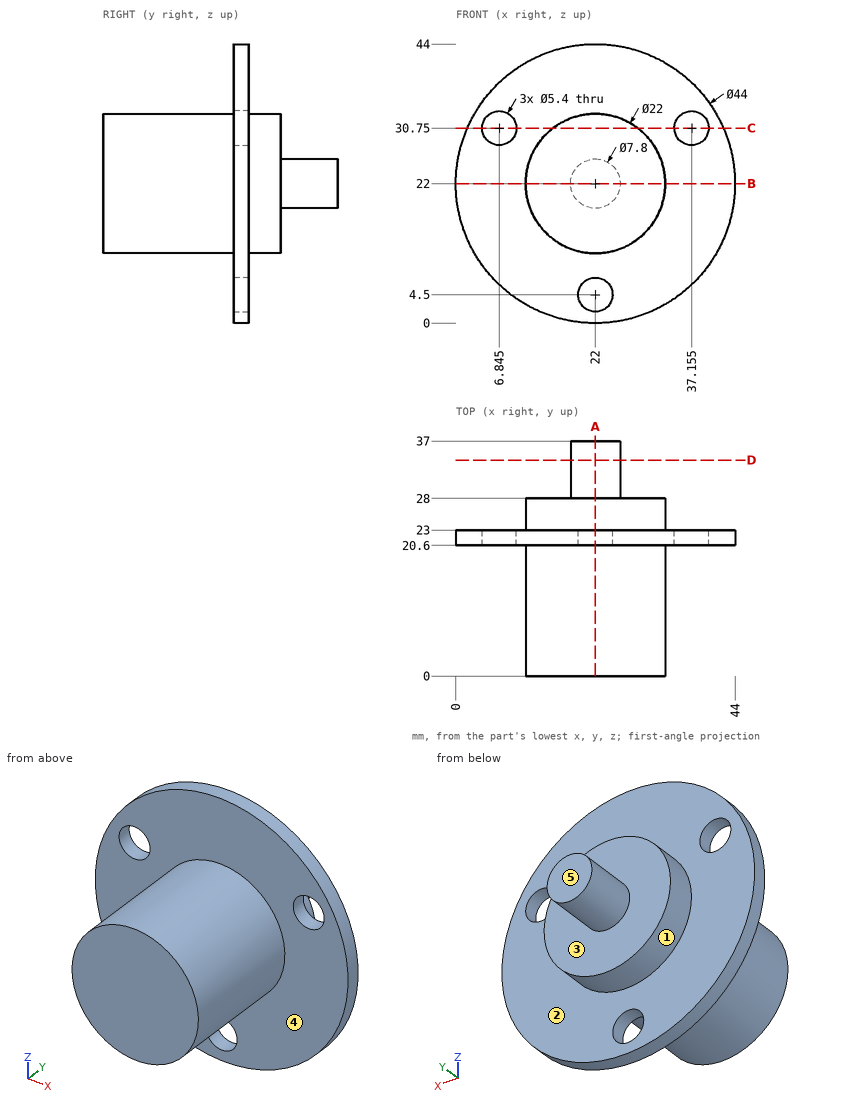
Check sheet for the drawn part. Datum: minimum x, y, z corner. Units: mm. A direction names the side the tool comes from. Round coordinates to 2 decimals unless told otherwise and drop trailing zeros. Loops run counter-clockwise (first coordinate to the right, second up) from the corner with the lowest first, then second, coordinate; pieces in that order, holes last. Notation, with made-up numbers: (89, 31.25) -> (95, 31.25) arc R35 cw to (95, 69.25) -> close; hole circle Ø9 at (28, 48). An arc over 180 degrees is marked (long way). Put each result on its own line as item: value. Start each with the question number.
1. Scan lines: probe 1 along Y at (x, z) = (31, 21); probe 2 along X at (y, z) = (22.4, 30.75) (1 decimal); probe 3 along Y at (x, z) = (27.5, 35.5). Record each from-to range of solid material in increasing order.
2. Section check C-C (z = 30.75). Enter the section's corners in (x, y) (1 decimal), plus the area to 3 significant figures.
3. Gauge pin test, flat ends, axial feed: pin 1 (22 mm diameter, centred on x = 32, z = 15, fed in from +Y); pin 2 (1 mm diameter, centred on x = 34, z = 12, fed in from -Y); pin 3 (1 mm diameter, centred on x = 6.5, z = 7, fed in from +Y); pin 4 (12 mm diameter, centred on x = 32.5, y = 6.5, fed in from -Z). Record the tip position at first contact, or that the pin passes through.
4. Draft check along X on the marked faces 1 and 2. Enter one of: +X half, -X half, draft (parallel to the pull), parting line (faces both ways), or undercut.
5. Section check B-B (z = 22). Enter the section's corners in (x, y).
6. Section check A-A (x = 22). Enter the section's corners in (y, z), plus the area to 3 significant figures.
7. Section check D-D (y = 34). Enter the section's corners in (x, z), plus the area to 3 significant figures.
8. Access from +Z, -Z, +X, -X, +Y, -Y to the whole of each face (thin tool, end or side, straight path). Record for the marked faces 3, 4 and 5.
Findings:
1. probe 1: y = 0 to 28
1. probe 2: x = 1.8 to 4.1, 9.5 to 34.5, 39.9 to 42.2
1. probe 3: y = 20.6 to 23
2. outline: (1.8, 20.6) -> (4.1, 20.6) -> (4.1, 23) -> (1.8, 23) -> close; (9.5, 20.6) -> (15.3, 20.6) -> (15.3, 0) -> (28.7, 0) -> (28.7, 20.6) -> (34.5, 20.6) -> (34.5, 23) -> (28.7, 23) -> (28.7, 28) -> (15.3, 28) -> (15.3, 23) -> (9.5, 23) -> close; (39.9, 20.6) -> (42.2, 20.6) -> (42.2, 23) -> (39.9, 23) -> close
2. area: 412 mm^2
3. pin 1: stops at y = 37
3. pin 2: stops at y = 20.6
3. pin 3: stops at y = 23
3. pin 4: stops at z = 11.96
4. face 1: parting line
4. face 2: draft
5. outline: (0, 20.6) -> (11, 20.6) -> (11, 0) -> (33, 0) -> (33, 20.6) -> (44, 20.6) -> (44, 23) -> (33, 23) -> (33, 28) -> (25.9, 28) -> (25.9, 37) -> (18.1, 37) -> (18.1, 28) -> (11, 28) -> (11, 23) -> (0, 23) -> close
6. outline: (0, 11) -> (20.6, 11) -> (20.6, 7.2) -> (23, 7.2) -> (23, 11) -> (28, 11) -> (28, 18.1) -> (37, 18.1) -> (37, 25.9) -> (28, 25.9) -> (28, 33) -> (23, 33) -> (23, 44) -> (20.6, 44) -> (20.6, 33) -> (0, 33) -> close; (20.6, 0) -> (23, 0) -> (23, 1.8) -> (20.6, 1.8) -> close
6. area: 726 mm^2
7. outline: circle Ø7.8 at (22, 22)
7. area: 47.8 mm^2
8. face 3: +Y
8. face 4: -Y
8. face 5: +Z, -Z, +X, -X, +Y
